```python
from build123d import *

# Parameters (mm, degrees)
SKETCH_1_W      = 20
SKETCH_1_H      = 6
SKETCH_1_R      = 1.5
EXTRUDE_1_DEPTH = 5
SKETCH_2_R      = 1.5
SKETCH_2_R_2    = 5.25
EXTRUDE_2_DEPTH = 5


with BuildPart() as part:
    # 草图1 → 凸台-拉伸1 (new body)
    with BuildSketch(Plane(origin=(0, 0, 0), x_dir=(0, 0, -1), z_dir=(1, 0, 0))):
        with Locations((10, 3)):
            Rectangle(SKETCH_1_W, SKETCH_1_H)
        with Locations((5, 3)):
            Circle(SKETCH_1_R, mode=Mode.SUBTRACT)
        with Locations((15, 3)):
            Circle(SKETCH_1_R, mode=Mode.SUBTRACT)
    extrude(amount=EXTRUDE_1_DEPTH)

    # 草图2 → 凸台-拉伸2 (add)
    # profile 1 of 2: a face of its own
    with BuildSketch(Plane.XY):
        with BuildLine():
            ThreePointArc((0, 0), (-2.514718626, -7), (0, -14))
            Line((0, -14), (16.970562748, -14))
            ThreePointArc((16.970562748, -14), (19.485281374, -7), (16.970562748, 0))
            Line((16.970562748, 0), (0, 0))
        make_face()
        with Locations((0.485281374, -7)):
            Circle(SKETCH_2_R, mode=Mode.SUBTRACT)
        with Locations((8.485281374, -7)):
            Circle(SKETCH_2_R_2, mode=Mode.SUBTRACT)
        with Locations((16.485281374, -7)):
            Circle(SKETCH_2_R, mode=Mode.SUBTRACT)
    # profile 2 of 2: a face of its own
    with BuildSketch(Plane.XY):
        Polygon((0, 6), (0, 0), (16.970562748, 0), (5, 6), align=None)
    extrude(amount=EXTRUDE_2_DEPTH)


solid = part.part
```
Design review of the part built by this model. Coordinates are the model's own, in mm. A direction names the side the tool comes from. Coordinates: 2 decimals unless noted, no trailing zeros. Loops run counter-clockwise (first coordinate to the right, second up) from the corner with the lowest first, then second, coordinate; pieces in that order, holes last. Notation, with made-up numbers: (42.5, -3.5) - (88.5, -3.5) arc R18 cw to (88.5, 13.5) - close; hole circle Ø8 at (71.25, 9.25). An arc over 180 degrees is marked (long way). Use CSV: the item, a comma, the result in double quotes. Start each with the question number.
1) Wall thickness on L1, parallel to Y at x = 3.9, z = -5; L2, parallel to Z at x = 17.75, y = -11; L3, parallel to Y at x = 1.75, z = -1: over which ranges is each line inside the solid? List them lowest first. Write a range as from..to.
2) Consider section B-B on y = -3.75. Write out the cut boundary in (x, z).
3) Tool access review of faces 1 (the flat face through (5, 3, -10)), 2 (the flat face through (0, 3, -8)), 3 (the flat face through (2, 0, -10)): name each direction out of +Z, -Z, +X, -X, +Y, -Y from which nothing blocks a thin tool from reaching the whole face with its end or side.
4) Consider section C-C on y = -7. Write out the cut boundary in (x, z), then the cut area to 3 significant figures.
5) The part is to be moulded in two halves that separate along Y. For faces 4 (the flat face through (8, -14, 2)), 5 (the cylindrical face through (0.16, -8.464, 2.465)), 6 (the flat face through (2, 3, -20)), say which applies: +Y half, -Y half, draft (parallel to the pull), parting line (faces both ways), or undercut.
6) For pin 1 Ø3 at (y, z) = (3, -9) entering from +X; pin 2 Ø1.5 at (x, y) = (2, -11.5) entering from -Z; pin 3 Ø4 at (x, z) = (2, -9.5) entering from -Y, all flat-tipped, find the tip position at first contact; note any pin that passes through.
7) Consider section A-A on z = -15. Write out the cut boundary in (x, y).
8) Consider section D-D on y = 3. Write out the cut boundary in (x, z).
Geometry says:
1,L1,"0..1.5, 4.5..6"
1,L2,"0..5"
1,L3,"0..6"
2,outline,"(-2.02, 0) - (4.36, 0) - (4.36, 5) - (-2.02, 5) - close; (12.61, 0) - (18.99, 0) - (18.99, 5) - (12.61, 5) - close"
3,face 1,"-Z, +X, +Y, -Y"
3,face 2,"+Z, -Z, -X, +Y"
3,face 3,"-Z, +X, -X, -Y"
4,outline,"(-2.51, 0) - (-1.01, 0) - (-1.01, 5) - (-2.51, 5) - close; (1.99, 0) - (3.24, 0) - (3.24, 5) - (1.99, 5) - close; (13.74, 0) - (14.99, 0) - (14.99, 5) - (13.74, 5) - close; (17.99, 0) - (19.49, 0) - (19.49, 5) - (17.99, 5) - close"
4,area,"27.5 mm^2"
5,face 4,"-Y half"
5,face 5,"undercut"
5,face 6,"draft"
6,pin 1,"x = 5"
6,pin 2,"z = 0"
6,pin 3,"y = 0"
7,outline,"(0, 0) - (5, 0) - (5, 1.5) - (0, 1.5) - close; (0, 4.5) - (5, 4.5) - (5, 6) - (0, 6) - close"
8,outline,"(0, -20) - (5, -20) - (5, -16.5) - (0, -16.5) - close; (0, -13.5) - (5, -13.5) - (5, -6.5) - (0, -6.5) - close; (0, -3.5) - (5, -3.5) - (5, 0) - (10.99, 0) - (10.99, 5) - (0, 5) - close"
